Print and shaded views of the part. All mm, measured from the part's lowest x, y and z. Round coordinates to 2 decimals unless told otherwise and drop trailing zeros. Order: outer loops, then holes, each group sorted by start corner. A loop starts at its lowest first (then second) coordinate and runs counter-clockwise, first axis right, second up. Notation, with made-up numbers: (30, 83.5) -> (48, 83.5) arc R28 ccw to (48, 120.5) -> close; hole circle Ø2 at (78.25, -7). An arc over 180 degrees is marked (long way). Answer as CSV lines item,"result".
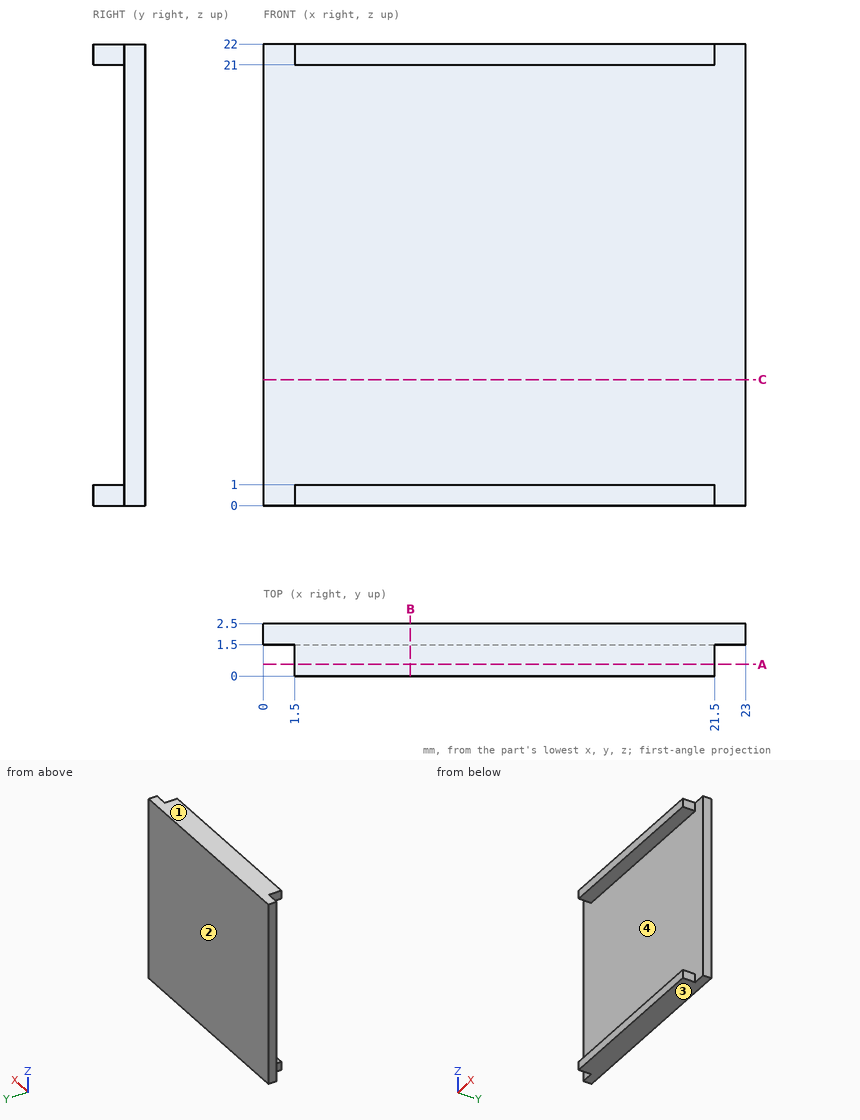
Q1. Flat gauge pins, fed straight in: pin 1 (2 mm diameter, centred on x = 17.5, z = 16, fed in from -Y); pin 2 (0.5 mm diameter, centred on y = 0.5, z = 21.5, fed in from +X); pin 3 (0.5 mm diameter, centred on y = 0.5, z = 0.5, fed in from -X). Where does each tip first touch, or does it go through?
Checks:
pin 1,"y = 1.5"
pin 2,"x = 21.5"
pin 3,"x = 1.5"
Q2. Saw through at B-B (x = 7). Write the cut outline in (y, z), plus the area to 3 significant figures.
Checks:
outline,"(0, 0) -> (2.5, 0) -> (2.5, 22) -> (0, 22) -> (0, 21) -> (1.5, 21) -> (1.5, 1) -> (0, 1) -> close"
area,"25.0 mm²"
Q3. Saw through at C-C (z = 6). Write the cut outline in (x, y).
Checks:
outline,"(0, 1.5) -> (23, 1.5) -> (23, 2.5) -> (0, 2.5) -> close"
Q4. Wall check: L1, parallel to Z at x = 9.75, y = 0.35; L2, parallel to Y at x = 10, z = 7. Give the ranges that are in metal, low to high. Write a range as [from, to].
Checks:
L1,"[0, 1], [21, 22]"
L2,"[1.5, 2.5]"
Q5. Saw through at A-A (y = 0.55). Write the cut outline in (x, z).
Checks:
outline,"(1.5, 0) -> (21.5, 0) -> (21.5, 1) -> (1.5, 1) -> close; (1.5, 21) -> (21.5, 21) -> (21.5, 22) -> (1.5, 22) -> close"
Q6. Mould opens along Z. For the marked faces 1, 2, 3 and 4 say: +Z half, -Z half, draft (parallel to the pull), parting line (faces both ways), or undercut.
Checks:
face 1,"+Z half"
face 2,"draft"
face 3,"-Z half"
face 4,"undercut"
